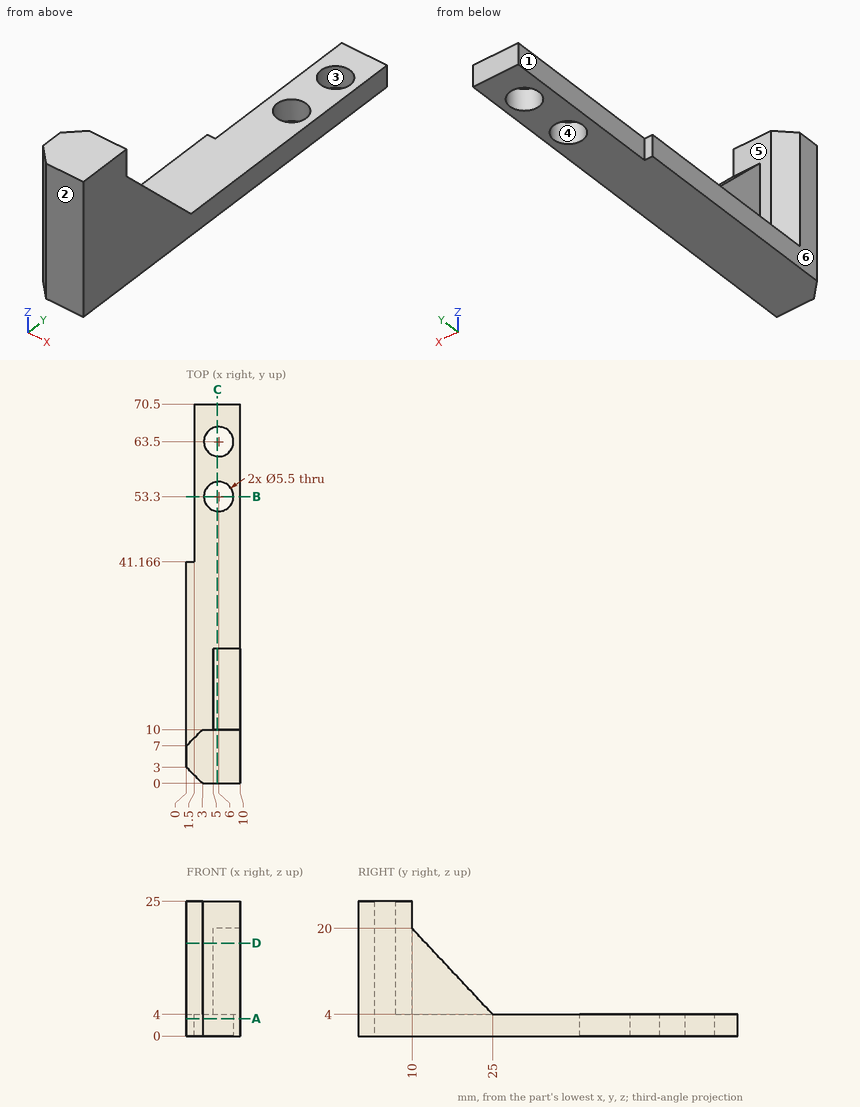
Design review of the part shown in the three views and the two pictorial views. Dimensions are in mm from the part's minimum x, y and z. A direction names the side the tool comes from. Round coordinates to 2 decimals unless told otherwise and drop trailing zeros. Loops run counter-clockwise (first coordinate to the right, second up) from the corner with the lowest first, then second, coordinate; pieces in that order, holes last.
Q1. Add section D-D on z = 17.25. Write out the cut boundary in (x, y).
Result sheet:
outline: (0, 3) - (3, 0) - (10, 0) - (10, 12.58) - (5, 12.58) - (5, 10) - (3, 10) - (0, 7) - close
Q2. Insertion check: pin 1 Ø2 at (x, y) = (5.5, 23.5) entering from +Z; pin 2 Ø2 at (y, z) = (53.5, 2) entering from -X; pin 3 Ø3.5 at (x, z) = (7.5, 11) entering from +Y. Each pin has a flat end and moves straight along its axis. Give the tip position at first contact, or say it passes through.
Result sheet:
pin 1: stops at z = 6.67
pin 2: stops at x = 1.5
pin 3: stops at y = 20.08
Q3. Add section A-A on z = 3.25. Write out the cut boundary in (x, y), plus the area to 3 significant figures.
Result sheet:
outline: (0, 3) - (3, 0) - (10, 0) - (10, 70.5) - (1.5, 70.5) - (1.5, 41.17) - (0, 41.17) - close; hole circle Ø5.5 at (6, 53.3); hole circle Ø5.5 at (6, 63.5)
area: 609 mm2
Q4. Machinability: for the marked faces 5 and 6, which of the approach directions +Z, -Z, +X, -X, +Y, -Y give a long, thin tool a straight path to every point of the face, cutting with its end or side? Answer none if there is none.
Result sheet:
face 5: +Z, -X, +Y
face 6: +Z, -Z, -X, +Y, -Y
Q5. Add section C-C on x = 5.75. Write out the cut boundary in (y, z), plus the area to 3 significant figures.
Result sheet:
outline: (0, 0) - (50.56, 0) - (50.56, 4) - (25, 4) - (10, 20) - (10, 25) - (0, 25) - close; (56.04, 0) - (60.76, 0) - (60.76, 4) - (56.04, 4) - close; (66.24, 0) - (70.5, 0) - (70.5, 4) - (66.24, 4) - close
area: 568 mm2
Q6. Add section B-B on y = 53.3. Write out the cut boundary in (x, z), plus the area to 3 significant figures.
Result sheet:
outline: (1.5, 0) - (3.25, 0) - (3.25, 4) - (1.5, 4) - close; (8.75, 0) - (10, 0) - (10, 4) - (8.75, 4) - close
area: 12.0 mm2
Q7. Mouldability with a two-part tool opening along X and no side actions: class the marked faces 1, 2, 3 and 4 as +X half, -X half, draft (parallel to the pull), parting line (faces both ways), or undercut.
Result sheet:
face 1: -X half
face 2: draft
face 3: undercut
face 4: undercut
Q8. To check wall thickness, follow line 1 along Y through (x, z) = (6, 1.6); line 2 along Z through (x, y) = (8.75, 61); line 3 along Y through (x, z) = (4.25, 22). State the ranges of each line that lie inside material, in increasing order.
Result sheet:
line 1: y = 0 to 50.55, 56.05 to 60.75, 66.25 to 70.5
line 2: z = 0 to 4
line 3: y = 0 to 10
